Model file for the job. Use its own axes, mm. Face numbers are marked on the shaded views. A direction names the side the tool comes from. Give positions to 0.01 mm unless a question says otherwise; leave off trailing zeros. Order: outer loops, then holes, each group sorted by start corner. A loop starts at its lowest first (then second) coordinate and runs counter-clockwise, first axis right, second up. Notation, with made-up numbers: (59, -21) - (68, -21) arc R34 cw to (68, 17) - close; hole circle Ø5 at (-10.75, -12.5). An arc over 180 degrees is marked (long way). Use CSV: the item, a comma, the result in double quotes. Start each with the question number.
(1) Band-saw the part on C-C, the plane x = 0. Give the cut face in (y, z), then the cut area to 3 significant figures.
(2) Probe L1, parallel to Z at x = 0, y = -12; L2, parallel to Y at x = -40, z = -38; L3, parallel to Y at x = 46, z = 17.5. List the from-to ranges inside material, lowest first.
(3) Band-saw the part on A-A, the plane y = -22. Give the cut face in (x, z), then the cut area to 3 significant figures.
(4) Band-saw the part on D-D, the plane y = -8. Give the cut face in (x, z), then the cut area to 3 significant figures.
(5) Tool access for the marked faces 5 and 6: list every direction of +Z, -Z, +X, -X, +Y, -Y with a clear straight run to the whole face (end or side of a thin tool).
(6) Drop flat-ended pins along their axis: pin 1 Ø5 at (y, z) = (-25.5, -5.5) entering from +X; pin 2 Ø4 at (x, z) = (-20, -26.5) entering from -Y; pin 3 Ø13 at (x, z) = (-11, 4) entering from -Y. Give the stop position or say it passes through.
(7) Pull direction X, two halves, no side cores. Call the marked faces 1, 2, 3 and 4: +X half, -X half, draft (parallel to the pull), parting line (faces both ways), or undercut.
(8) Band-saw the part on B-B, the plane z = 0. Give the cut face in (x, y).
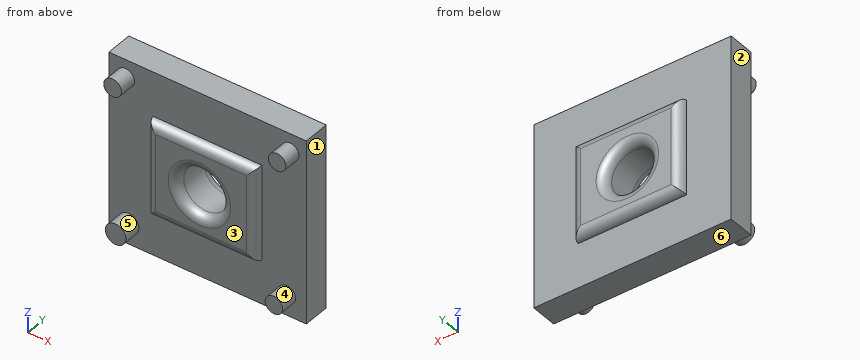
from build123d import *

# Parameters (mm, degrees)
F0_W     = 61.9982723147
F0_H     = 54.2247854173
F0_R     = 12.7819973787
F1_DEPTH = 25.4
F2_R     = 5.08
F3_DEPTH = 25.4
F4_DEPTH = 25.4
F5_DEPTH = 25.4
F6_DEPTH = 25.4
F7_R     = 5.0618882288
F7_R_2   = 4.9888661586
F7_R_3   = 4.9841843595
F7_R_4   = 5.8719562736
F8_DEPTH = 10


with BuildPart() as f1:
    # F0 (on Front) → F1 (new body)
    with BuildSketch(Plane.XZ):
        with Locations((0.8531874046, 0.758389011)):
            Rectangle(F0_W, F0_H)
        Circle(F0_R, mode=Mode.SUBTRACT)
    extrude(amount=F1_DEPTH)

    # F2
    f2_edges = [f1.edges().sort_by_distance(p)[0] for p in [
        (0.853187, -25.4, 27.870782),
        (-30.145949, -25.4, 0.758389),
        (0.853187, -25.4, -26.354004),
        (31.852324, -25.4, 0.758389),
        (-12.781997, -25.4, 0),
        (0.853187, 0, 27.870782),
        (-30.145949, 0, 0.758389),
        (0.853187, 0, -26.354004),
        (31.852324, 0, 0.758389),
        (-12.781997, 0, 0),
    ]]
    fillet(f2_edges, radius=F2_R)

    # F3 (add): a face of the model
    f3_faces = [f1.faces().sort_by_distance(p)[0] for p in [
        (0.8531874046, -12.7, 27.8707817197),
    ]]
    extrude(f3_faces, amount=F3_DEPTH)

    # F4 (add): a face of the model
    f4_faces = [f1.faces().sort_by_distance(p)[0] for p in [
        (0.8531874046, -12.7, -26.3540036976),
    ]]
    extrude(f4_faces, amount=F4_DEPTH)

    # F5 (add): a face of the model
    f5_faces = [f1.faces().sort_by_distance(p)[0] for p in [
        (-30.1459487528, -12.7, 0.758389011),
    ]]
    extrude(f5_faces, amount=F5_DEPTH)

    # F6 (add): a face of the model
    f6_faces = [f1.faces().sort_by_distance(p)[0] for p in [
        (31.8523235619, -12.7, 0.758389011),
    ]]
    extrude(f6_faces, amount=F6_DEPTH)

    # F7 (on face) → F8 (join)
    with BuildSketch(Plane.XZ.offset(20.32)):
        with Locations((-45.9536351264, 43.1434102356)):
            Circle(F7_R)
        with Locations((48.043269664, 42.9407022893)):
            Circle(F7_R_2)
        with Locations((46.2194345891, -39.781190455)):
            Circle(F7_R_3)
        with Locations((-44.2356690764, -40.0870218873)):
            Circle(F7_R_4)
    extrude(amount=F8_DEPTH)


solid = f1.part
Answer block:
1,outline,"(-25.4, -21.27) arc R5.08 ccw to (-20.32, -26.35) - (-20.32, -51.75) - (-5.08, -51.75) - (-5.08, -26.35) arc R5.08 ccw to (0, -21.27) - (0, -17.86) arc R5.08 ccw to (-5.08, -12.78) - (-20.32, -12.78) arc R5.08 ccw to (-25.4, -17.86) - close; (-25.4, 17.86) arc R5.08 ccw to (-20.32, 12.78) - (-5.08, 12.78) arc R5.08 ccw to (0, 17.86) - (0, 22.79) arc R5.08 ccw to (-5.08, 27.87) - (-5.08, 53.27) - (-20.32, 53.27) - (-20.32, 27.87) arc R5.08 ccw to (-25.4, 22.79) - close"
1,area,"1,460 mm2"
2,L1,"z = -51.75 to -12.78, 12.78 to 53.27"
2,L2,"y = -30.32 to -5.08"
2,L3,"y = -20.32 to -5.08"
3,outline,"circle Ø10.12 at (-45.95, 43.14); circle Ø11.74 at (-44.24, -40.09); (-29.86, -26.07) - (31.57, -26.07) - (31.57, 27.58) - (-29.86, 27.58) - close; circle Ø9.97 at (46.22, -39.78); circle Ø9.98 at (48.04, 42.94); hole circle Ø26.14 at (0, 0)"
3,area,"3,100 mm2"
4,outline,"(-55.55, -51.75) - (57.25, -51.75) - (57.25, 53.27) - (-55.55, 53.27) - close; hole circle Ø25.56 at (0, 0)"
4,area,"11,300 mm2"
5,face 5,"-Y"
5,face 6,"-Z, +X, -X, +Y, -Y"
6,pin 1,"stops at x = 31.09"
6,pin 2,"stops at y = -24.24"
6,pin 3,"stops at y = -25.4"
7,face 1,"+X half"
7,face 2,"-X half"
7,face 3,"draft"
7,face 4,"undercut"
8,outline,"(-55.55, -20.32) - (-30.15, -20.32) arc R5.08 ccw to (-25.07, -25.4) - (-17.86, -25.4) arc R5.08 ccw to (-12.78, -20.32) - (-12.78, -5.08) arc R5.08 ccw to (-17.86, 0) - (-25.07, 0) arc R5.08 ccw to (-30.15, -5.08) - (-55.55, -5.08) - close; (12.78, -20.32) arc R5.08 ccw to (17.86, -25.4) - (26.77, -25.4) arc R5.08 ccw to (31.85, -20.32) - (57.25, -20.32) - (57.25, -5.08) - (31.85, -5.08) arc R5.08 ccw to (26.77, 0) - (17.86, 0) arc R5.08 ccw to (12.78, -5.08) - close"
